from build123d import *

# Parameters (mm, degrees)
EXTRUDE_1_DEPTH          = 350
EXTRUDE_2_DEPTH          = 1
EXTRUDE_2_DEPTH_BACK     = 5
CUT_EXTRUDE_1_DEPTH      = 360.210404844
CUT_EXTRUDE_1_DEPTH_BACK = 360.210404844
SKETCH_4_OUTSIDE_W       = 161.658
SKETCH_4_OUTSIDE_H       = 471.658


with BuildPart() as part:
    # 草图2 → 凸台-拉伸1 (new body)
    with BuildSketch(Plane.XY):
        with BuildLine():
            Line((80, -10.494126695), (80, -6.44149283))
            ThreePointArc((80, -6.44149283), (40.129455609, -1.612974895), (0, 0))
            Line((0, 0), (0, -4))
            ThreePointArc((0, -4), (40.131576351, -5.626197519), (80, -10.494126695))
        make_face()
    extrude(amount=EXTRUDE_1_DEPTH)

    # 草图3 → 凸台-拉伸2 (add, two sides: drawn at the far end of the back side and taken through both)
    with BuildSketch(Plane(origin=(0, 0, 0), x_dir=(1, 0, 0), z_dir=(0, 1, 0)).offset(-EXTRUDE_2_DEPTH_BACK)):
        with BuildLine():
            Line((0, 0), (0, 20))
            ThreePointArc((0, 20), (20, 40), (40, 20))
            Line((40, 20), (40, 0))
            Line((40, 0), (0, 0))
        make_face()
    extrude(amount=EXTRUDE_2_DEPTH + EXTRUDE_2_DEPTH_BACK)

    # 草图4 outside → 切除-拉伸1 (cut, two sides: drawn at the far end of the back side and taken through both)
    with BuildSketch(Plane(origin=(0, 1, 0), x_dir=(1, 0, 0), z_dir=(0, 1, 0)).offset(-CUT_EXTRUDE_1_DEPTH_BACK)):
        with Locations((40, -155)):
            Rectangle(SKETCH_4_OUTSIDE_W, SKETCH_4_OUTSIDE_H)
        with BuildLine():
            Line((0, -350), (20, -350))
            ThreePointArc((20, -350), (32.037873221, -232.445661311), (67.651801878, -119.770992366))
            ThreePointArc((67.651801878, -119.770992366), (73.805604709, -91.100068227), (68.49542517, -62.260977161))
            ThreePointArc((68.49542517, -62.260977161), (55.031874412, -30.771595648), (40, 0))
            Line((40, 0), (40, 103.702750203))
            Line((40, 103.702750203), (-64.531778678, 103.702750203))
            Line((-64.531778678, 103.702750203), (-64.531778678, -350))
            Line((-64.531778678, -350), (0, -350))
        make_face(mode=Mode.SUBTRACT)
    extrude(amount=CUT_EXTRUDE_1_DEPTH + CUT_EXTRUDE_1_DEPTH_BACK, mode=Mode.SUBTRACT)


solid = part.part
Can you work these out from the model? Positions are in its coordinate system, mm. A direction names the side the tool comes from. Give positions to 0.01 mm unless a question says otherwise; leave off trailing zeros. Order: outer loops, then holes, each group sorted by start corner. A loop starts at its lowest first (then second) coordinate and runs counter-clockwise, first axis right, second up. Notation, with made-up numbers: M -17.5,9 L -1.5,9 A27 ccw -1.5,36 Z; hole C 46.25,-8.75 d4. An arc over 180 degrees is marked long. Use a Markdown table: item, result. Add a question column.
Item 1: Will these pins go through, and if not, where does the flat tip stop? pin 1 (2 mm diameter, centred on x = 20.5, z = 193.5, fed in from +Y); pin 2 (1 mm diameter, centred on y = -5.5, z = 57, fed in from +X); pin 3 (6 mm diameter, centred on x = 24, y = -3.5, fed in from -Z) (3 decimals); pin 4 (2 mm diameter, centred on x = 16.5, y = 0, fed in from +Z).
Item 2: If I drill on L1, parallel to Y at x = 42.5, z = 50.5; L2, parallel to X at y = -2.25, z = -22.5; L3, parallel to Y at x = 8, z = 182.5, over which ranges is the centre line in solid material (lowest first)? Write a range as [from, to].
Item 3: Suppose I cut it at A-A (z = 311.5). List the corners of the cut face in (x, y) for me.
Item 4: Suppose I cut it at B-B (x = 47). List the corners of the cut face in (y, z) for me.
Item 5: For faces 1 (the flat face through (20, -5, -20)), 2 (the cylindrical face through (28.278, -4.807, 133.661)), 3 (the flat face through (40, -2, -10)), which set-ups out of +Z, -Z, +X, -X, +Y, -Y let a thin tool reach every point of the face, with its end or its side?
Answer sheet:
| question | item | result |
|---|---|---|
| 1 | pin 1 | stops at y = -0.38 |
| 1 | pin 2 | stops at x = 66.58 |
| 1 | pin 3 | stops at z = -39.975 |
| 1 | pin 4 | stops at z = 350 |
| 2 | L1 | y = [-5.82, -1.81] |
| 2 | L2 | x = [0.16, 39.84] |
| 2 | L3 | y = [-4.06, -0.06] |
| 3 | outline | M 0,-4 A496 cw 21.28,-4.46 L 21.28,-0.45 A500 ccw 0,0 Z |
| 4 | outline | M -6.23,13.84 L -2.21,13.84 L -2.21,175.1 L -6.23,175.1 Z |
| 5 | face 1 | -Z, +X, -X, -Y |
| 5 | face 2 | +Z, -X, -Y |
| 5 | face 3 | -Z, +X, +Y, -Y |
